Geometry check sheet. Reference: the model listing, model coordinates, mm. Face numbers are marked on the shaded views. A direction names the side the tool comes from. Give positions to 0.01 mm unless a question says otherwise; leave off trailing zeros. Order: outer loops, then holes, each group sorted by start corner. A loop starts at its lowest first (then second) coordinate and runs counter-clockwise, first axis right, second up.
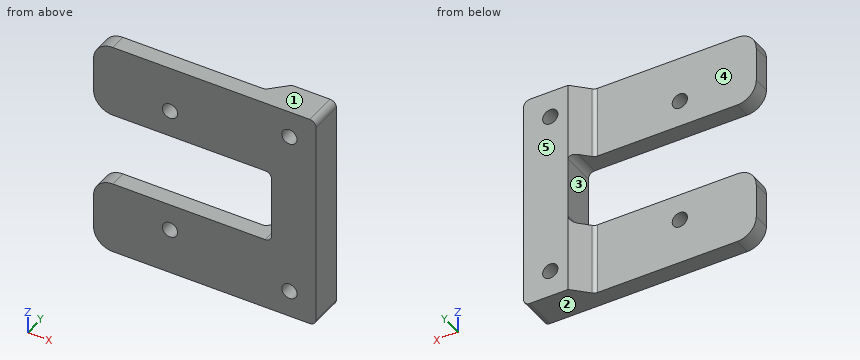
```python
from build123d import *

# Parameters (mm, degrees)
SKETCH1_W           = 7
SKETCH1_H           = 2.635
BOSS_EXTRUDE1_DEPTH = 17.2
CUT_EXTRUDE1_REACH  = 41.352
SKETCH2_R           = 1.2
CUT_EXTRUDE2_REACH  = 41.087
SKETCH3_R           = 1.2
SKETCH3_W           = 28
SKETCH3_H           = 11.6
CHAMFER1_SIZE       = 2.635
FILLET2_R           = 1
FILLET3_R           = 3
FILLET4_R           = 1


with BuildPart() as part:
    # Sketch1 → Boss-Extrude1 (new, symmetric)
    with BuildSketch(Plane.XY):
        Polygon((0, -5.27), (0, -2.635), (-7, -2.635), (-35, -2.635), (-35, -5.27), align=None)
        with Locations((-3.5, -1.3175)):
            Rectangle(SKETCH1_W, SKETCH1_H)
    extrude(amount=BOSS_EXTRUDE1_DEPTH, both=True)

    # Sketch2 → Cut-Extrude1 (cut, up to next)
    with BuildSketch(Plane(origin=(0, 0, 0), x_dir=(1, 0, 0), z_dir=(0, 1, 0)), mode=Mode.PRIVATE) as cut_extrude1_sk1:
        with Locations(Location((-4.2, 13, 0), (0, 0, 270))):
            Circle(SKETCH2_R)
    cut_extrude1_tool1 = extrude(cut_extrude1_sk1.sketch, amount=-CUT_EXTRUDE1_REACH, mode=Mode.PRIVATE) & part.part
    # Sketch2 → Cut-Extrude1 (cut, up to next)
    with BuildSketch(Plane(origin=(0, 0, 0), x_dir=(1, 0, 0), z_dir=(0, 1, 0)), mode=Mode.PRIVATE) as cut_extrude1_sk2:
        with Locations(Location((-4.2, -13, 0), (0, 0, 270))):
            Circle(SKETCH2_R)
    cut_extrude1_tool2 = extrude(cut_extrude1_sk2.sketch, amount=-CUT_EXTRUDE1_REACH, mode=Mode.PRIVATE) & part.part
    add(cut_extrude1_tool1.solids().sort_by_distance((-4.2, 0, -13))[0], mode=Mode.SUBTRACT)
    add(cut_extrude1_tool2.solids().sort_by_distance((-4.2, 0, 13))[0], mode=Mode.SUBTRACT)

    # Sketch3 → Cut-Extrude2 (cut, up to next)
    with BuildSketch(Plane(origin=(0, -2.635, 0), x_dir=(1, 0, 0), z_dir=(0, 1, 0)), mode=Mode.PRIVATE) as cut_extrude2_sk1:
        with Locations(Location((-22.979761, 10, 0), (0, 0, 180))):
            Circle(SKETCH3_R)
    cut_extrude2_tool1 = extrude(cut_extrude2_sk1.sketch, amount=-CUT_EXTRUDE2_REACH, mode=Mode.PRIVATE) & part.part
    # Sketch3 → Cut-Extrude2 (cut, up to next)
    with BuildSketch(Plane(origin=(0, -2.635, 0), x_dir=(1, 0, 0), z_dir=(0, 1, 0)), mode=Mode.PRIVATE) as cut_extrude2_sk2:
        with Locations(Location((-22.979761, -10, 0), (0, 0, 180))):
            Circle(SKETCH3_R)
    cut_extrude2_tool2 = extrude(cut_extrude2_sk2.sketch, amount=-CUT_EXTRUDE2_REACH, mode=Mode.PRIVATE) & part.part
    # Sketch3 → Cut-Extrude2 (cut, up to next)
    with BuildSketch(Plane(origin=(0, -2.635, 0), x_dir=(1, 0, 0), z_dir=(0, 1, 0)), mode=Mode.PRIVATE) as cut_extrude2_sk3:
        with Locations((-21, 0)):
            Rectangle(SKETCH3_W, SKETCH3_H)
    cut_extrude2_tool3 = extrude(cut_extrude2_sk3.sketch, amount=-CUT_EXTRUDE2_REACH, mode=Mode.PRIVATE) & part.part
    add(cut_extrude2_tool1.solids().sort_by_distance((-22.979761, -2.635, -10))[0], mode=Mode.SUBTRACT)
    add(cut_extrude2_tool2.solids().sort_by_distance((-22.979761, -2.635, 10))[0], mode=Mode.SUBTRACT)
    add(cut_extrude2_tool3.solids().sort_by_distance((-21, -2.635, 0))[0], mode=Mode.SUBTRACT)

    # Chamfer1
    # the kernel refuses this chamfer: 2.635 mm, written as the material it adds along each edge
    with BuildSketch(Plane(origin=(-7, -2.635, 5.8), x_dir=(0.027495876610586358, 0.9996219169112968, 0), z_dir=(0, 0, 1))) as chamfer1_piece_1_section:
        Polygon((CHAMFER1_SIZE * 0.999621916911, CHAMFER1_SIZE * 0.0274958766106), (-CHAMFER1_SIZE * 0.0274958766106, CHAMFER1_SIZE * 0.999621916911), (0, 0), align=None)
    chamfer1_piece_1 = extrude(amount=11.4, mode=Mode.PRIVATE)
    chamfer1_piece_1 = split(chamfer1_piece_1, bisect_by=Plane(origin=(-7.870614947, 0, 11.5), z_dir=(0, -1, 0)), keep=Keep.TOP, mode=Mode.PRIVATE)
    add(chamfer1_piece_1)
    with BuildSketch(Plane(origin=(-7, -2.635, -17.2), x_dir=(0.027495876610586358, 0.9996219169112968, 0), z_dir=(0, 0, 1))) as chamfer1_piece_2_section:
        Polygon((CHAMFER1_SIZE * 0.999621916911, CHAMFER1_SIZE * 0.0274958766106), (-CHAMFER1_SIZE * 0.0274958766106, CHAMFER1_SIZE * 0.999621916911), (0, 0), align=None)
    chamfer1_piece_2 = extrude(amount=11.4, mode=Mode.PRIVATE)
    chamfer1_piece_2 = split(chamfer1_piece_2, bisect_by=Plane(origin=(-7.870614947, 0, -11.5), z_dir=(0, -1, 0)), keep=Keep.TOP, mode=Mode.PRIVATE)
    add(chamfer1_piece_2)

    # Fillet2
    fillet2_edges = [part.edges().sort_by_distance(p)[0] for p in [
        (-7, -2.635, -5.8),
        (-7, -2.635, 5.8),
        (-9.635, -2.635, 11.5),
        (-9.635, -2.635, -11.5),
    ]]
    fillet(fillet2_edges, radius=FILLET2_R)

    # Fillet3
    fillet3_edges = [part.edges().sort_by_distance(p)[0] for p in [
        (-35, -3.9525, -17.2),
        (-35, -3.9525, 17.2),
        (-35, -3.9525, 5.8),
        (-35, -3.9525, -5.8),
    ]]
    fillet(fillet3_edges, radius=FILLET3_R)

    # Fillet4
    fillet4_edges = [part.edges().sort_by_distance(p)[0] for p in [
        (0, -2.635, 17.2),
        (0, -2.635, -17.2),
    ]]
    fillet(fillet4_edges, radius=FILLET4_R)


solid = part.part
```
Q1. Release check for a two-part mould opening along Z. For the marked faces 1, 2 and 3 record: pulls with the +Z half, pulls with the -Z half, needs draft (parallel to the pull), parting line crosses it, or undercut.
Q2. Access from +Z, -Z, +X, -X, +Y, -Y to the whole of each face (thin tool, end or side, straight path). Record for the marked faces 4 and 5.
Q3. Cross-section at D-D, the plane x = -25.5. Record the boundary of the cut face in (y, z) (3 decimals).
Q4. Thickness scan on L1, parallel to X at y = -4, z = -13; L2, parallel to Z at x = -9.5, y = -4.35; L3, parallel to X at y = -0.5, z = -4. Record the ranges inside material, lowest first.
Q5. Gauge pin test, flat ends, axial feed: P1, Ø3.5, axis at x = -27, z = -12.5, coming from the +Y side (3 decimals); P2, Ø3, axis at y = -4.5, z = -3.5, coming from the -X side. Record the tip position at first contact, or that the pin passes through.
Q6. Cross-section at C-C, the plane y = -4.6. Record the boundary of the cut face in (x, z), and give its area (3 significant figures).
Q7. Cross-section at A-A, the plane z = -13. Record the boundary of the cut face in (x, y) (3 decimals), and give its area (3 significant figures).
Q8. Cross-section at B-B, the plane x = -4.2. Record the boundary of the cut face in (y, z).
Answers follow:
1. face 1: pulls with the +Z half
1. face 2: pulls with the -Z half
1. face 3: undercut
2. face 4: +Z, -Z, -X, +Y
2. face 5: +Z, -Z, +X, -X, +Y
3. outline: (-5.27, -17.2) - (-2.635, -17.2) - (-2.635, -5.8) - (-5.27, -5.8) - close; (-5.27, 5.8) - (-2.635, 5.8) - (-2.635, 17.2) - (-5.27, 17.2) - close
4. L1: x = -35 to -5.4, -3 to 0
4. L2: z = -17.2 to -5.8, 5.8 to 17.2
4. L3: x = -7 to 0
5. P1: stops at y = -2.635
5. P2: stops at x = -7.02
6. outline: (-35, -14.2) arc R3 ccw to (-32, -17.2) - (-1, -17.2) arc R1 ccw to (0, -16.2) - (0, 16.2) arc R1 ccw to (-1, 17.2) - (-32, 17.2) arc R3 ccw to (-35, 14.2) - (-35, 8.8) arc R3 ccw to (-32, 5.8) - (-8, 5.8) arc R1 cw to (-7, 4.8) - (-7, -4.8) arc R1 cw to (-8, -5.8) - (-32, -5.8) arc R3 ccw to (-35, -8.8) - close; hole circle Ø2.4 at (-22.98, -10); hole circle Ø2.4 at (-22.98, 10); hole circle Ø2.4 at (-4.2, -13); hole circle Ø2.4 at (-4.2, 13)
6. area: 853 mm2
7. outline: (-35, -5.27) - (-5.4, -5.27) - (-5.4, 0) - (-7, 0) - (-9.342, -2.342) arc R1 cw to (-10.049, -2.635) - (-35, -2.635) - close; (-3, -5.27) - (0, -5.27) - (0, 0) - (-3, 0) - close
7. area: 102 mm2
8. outline: (-5.27, -17.2) - (0, -17.2) - (0, -14.2) - (-5.27, -14.2) - close; (-5.27, -11.8) - (0, -11.8) - (0, 11.8) - (-5.27, 11.8) - close; (-5.27, 14.2) - (0, 14.2) - (0, 17.2) - (-5.27, 17.2) - close
